Geometry check sheet. Reference: the model listing, model coordinates, mm. Face numbers are marked on the shaded views. A direction names the side the tool comes from. Coordinates: 2 decimals unless noted, no trailing zeros. Write each loop counter-clockwise with the first axis right and the second up, starting at its lowest first coordinate (ties: lowest second). Pieces come first, ordered by that corner, then holes. Notation, with made-up numbers: M 23,-30 L 62,-30 A22 ccw 62,-5 Z; hole C -27.75,45.5 d4. An arc over 180 degrees is marked long. Answer as a JSON object with one key per item and string values. Group by question number.
```python
from build123d import *

# Parameters (mm, degrees)
SKETCH_1_W          = 50
SKETCH_1_H          = 45
SKETCH_1_W_2        = 45
SKETCH_1_H_2        = 40
EXTRUDE_1_DEPTH     = 90
SKETCH_2_W          = 48.4
SKETCH_2_H          = 1.9
CUT_EXTRUDE_1_DEPTH = 36
SKETCH_3_R          = 13.5
CUT_EXTRUDE_2_DEPTH = 2.5
EXTRUDE_2_DEPTH     = 36
SKETCH_5_W          = 45
SKETCH_5_H          = 36
CUT_EXTRUDE_3_DEPTH = 50.2
CUT_EXTRUDE_4_DEPTH = 36
SKETCH_7_W          = 2.2
SKETCH_7_H          = 1.9
EXTRUDE_3_DEPTH     = 30
CHAMFER_1_SIZE      = 2.2
SKETCH_8_W          = 3.95
SKETCH_8_H          = 3.95
EXTRUDE_4_DEPTH     = 6
SKETCH_9_R          = 2.025
CUT_EXTRUDE_5_DEPTH = 5
SKETCH_10_W         = 3.95
SKETCH_10_H         = 5
SKETCH_10_H_2       = 7.5
SKETCH_10_H_3       = 3.95
EXTRUDE_5_DEPTH     = 6
CUT_EXTRUDE_START   = -5
SKETCH_11_R         = 2.025
CUT_EXTRUDE_6_DEPTH = 5
CHAMFER_2_SIZE      = 3.95
FILLET_1_R          = 1.2
CUT_EXTRUDE_7_REACH = 125.637


with BuildPart() as part:
    # 草圖1 → 填料-伸長1 (new body)
    with BuildSketch(Plane(origin=(0, 0, 0), x_dir=(1, 0, 0), z_dir=(0, 1, 0))):
        Rectangle(SKETCH_1_W, SKETCH_1_H)
        Rectangle(SKETCH_1_W_2, SKETCH_1_H_2, mode=Mode.SUBTRACT)
    extrude(amount=-EXTRUDE_1_DEPTH)

    # 草圖2 → 除料-伸長1 (cut)
    with BuildSketch(Plane(origin=(0, 0, 0), x_dir=(1, 0, 0), z_dir=(0, 1, 0))):
        with Locations((0, -14.05)):
            Rectangle(SKETCH_2_W, SKETCH_2_H)
    extrude(amount=-CUT_EXTRUDE_1_DEPTH, mode=Mode.SUBTRACT)

    # 草圖3 → 除料-伸長2 (cut)
    with BuildSketch(Plane.XY.offset(22.5)):
        with BuildLine():
            Line((-22.5, 0), (-22.5, -17.3))
            ThreePointArc((-22.5, -17.3), (-9, -3.8), (4.5, -17.3))
            Line((4.5, -17.3), (4.5, 0))
            Line((4.5, 0), (-22.5, 0))
        make_face()
        with Locations((-9, -17.3)):
            Circle(SKETCH_3_R)
    extrude(amount=-CUT_EXTRUDE_2_DEPTH, mode=Mode.SUBTRACT)

    # 草圖4 → 填料-伸長2 (add)
    with BuildSketch(Plane.XY.offset(22.5)):
        with BuildLine():
            Line((11, 0), (11, -17.3))
            ThreePointArc((11, -17.3), (5.142135624, -31.442135624), (-9, -37.3))
            Line((-9, -37.3), (-25, -37.3))
            Line((-25, -37.3), (-25, -90))
            Line((-25, -90), (25, -90))
            Line((25, -90), (25, 0))
            Line((25, 0), (11, 0))
        make_face()
    extrude(amount=EXTRUDE_2_DEPTH)

    # 草圖5 → 除料-伸長3 (cut)
    with BuildSketch(Plane(origin=(-25, -90, 58.5), x_dir=(1, 0, 0), z_dir=(0, -1, 0))):
        with Locations((25, -20.5)):
            Rectangle(SKETCH_5_W, SKETCH_5_H)
    extrude(amount=-CUT_EXTRUDE_3_DEPTH, mode=Mode.SUBTRACT)

    # 草圖6 → 除料-伸長4 (cut)
    with BuildSketch(Plane(origin=(0, 0, 20), x_dir=(-1, 0, 0), z_dir=(0, 0, -1))):
        with BuildLine():
            Line((-22.5, -2.5), (-22.5, -39.8))
            Line((-22.5, -39.8), (9, -39.8))
            ThreePointArc((9, -39.8), (-6.909902577, -33.209902577), (-13.5, -17.3))
            Line((-13.5, -17.3), (-13.5, -2.5))
            Line((-13.5, -2.5), (-22.5, -2.5))
        make_face()
    extrude(amount=-CUT_EXTRUDE_4_DEPTH, mode=Mode.SUBTRACT)

    # 草圖7 → 填料-伸長3 (add)
    with BuildSketch(Plane(origin=(0, -38.5, 0), x_dir=(1, 0, 0), z_dir=(0, 1, 0))):
        with Locations((-21.4, -14.05)):
            Rectangle(SKETCH_7_W, SKETCH_7_H)
    extrude(amount=-EXTRUDE_3_DEPTH)

    # 導角1
    chamfer_1_edges = [part.edges().sort_by_distance(p)[0] for p in [
        (-20.3, -38.5, 14.05),
        (-20.3, -68.5, 14.05),
    ]]
    chamfer(chamfer_1_edges, length=CHAMFER_1_SIZE - 0.0001)  # a hair under: the kernel refuses the full size

    # 草圖8 → 填料-伸長4 (add)
    with BuildSketch(Plane.XZ.offset(90)):
        with Locations((-20.525, 54.025)):
            Rectangle(SKETCH_8_W, SKETCH_8_H)
        with Locations((20.525, 54.025)):
            Rectangle(SKETCH_8_W, SKETCH_8_H)
        with Locations((20.525, -18.025)):
            Rectangle(SKETCH_8_W, SKETCH_8_H)
        with Locations((-20.525, -18.025)):
            Rectangle(SKETCH_8_W, SKETCH_8_H)
    extrude(amount=-EXTRUDE_4_DEPTH)

    # 草圖9 → 除料-伸長5 (cut)
    with BuildSketch(Plane.XZ.offset(90)):
        with Locations(Location((-21.775, 55.275, 0), (0, 0, 270))):
            Circle(SKETCH_9_R)
        with Locations(Location((21.775, 55.275, 0), (0, 0, 270))):
            Circle(SKETCH_9_R)
        with Locations(Location((-21.775, -19.275, 0), (0, 0, 270))):
            Circle(SKETCH_9_R)
        with Locations(Location((21.775, -19.275, 0), (0, 0, 270))):
            Circle(SKETCH_9_R)
    extrude(amount=-CUT_EXTRUDE_5_DEPTH, mode=Mode.SUBTRACT)

    # 草圖10 → 填料-伸長5 (add)
    with BuildSketch(Plane(origin=(0, 0, 0), x_dir=(1, 0, 0), z_dir=(0, 1, 0))):
        with Locations((20.525, -17.5)):
            Rectangle(SKETCH_10_W, SKETCH_10_H)
        with Locations((-20.525, -18.75)):
            Rectangle(SKETCH_10_W, SKETCH_10_H_2)
        with Locations((-20.525, 18.025)):
            Rectangle(SKETCH_10_W, SKETCH_10_H_3)
        with Locations((20.525, 18.025)):
            Rectangle(SKETCH_10_W, SKETCH_10_H_3)
    extrude(amount=-EXTRUDE_5_DEPTH)

    # 草圖11 → 除料-伸長6 (cut)
    with BuildSketch(Plane(origin=(0, 0, 0), x_dir=(1, 0, 0), z_dir=(0, 1, 0)).offset(CUT_EXTRUDE_START)):
        with Locations(Location((21.775, -18.225, 0), (0, 0, 270))):
            Circle(SKETCH_11_R)
        with Locations(Location((-21.775, -18.225, 0), (0, 0, 270))):
            Circle(SKETCH_11_R)
        with Locations(Location((21.775, 19.275, 0), (0, 0, 90))):
            Circle(SKETCH_11_R)
        with Locations(Location((-21.775, 19.275, 0), (0, 0, 90))):
            Circle(SKETCH_11_R)
    extrude(amount=CUT_EXTRUDE_6_DEPTH, mode=Mode.SUBTRACT)

    # 導角2
    chamfer_2_edges = [part.edges().sort_by_distance(p)[0] for p in [
        (-22.5, -6, 18.75),
        (22.5, -6, 17.5),
        (22.5, -6, -18.025),
        (-22.5, -6, -18.025),
    ]]
    chamfer(chamfer_2_edges, length=CHAMFER_2_SIZE - 0.0001)  # a hair under: the kernel refuses the full size

    # 圓角1
    fillet_1_edges = [part.edges().sort_by_distance(p)[0] for p in [
        (-18.55, -87, 52.05),
        (18.55, -87, 52.05),
        (18.55, -87, -16.05),
        (-18.55, -87, -16.05),
        (-18.55, -3, 15),
        (18.55, -3, 15),
        (-18.55, -3, -16.05),
        (18.55, -3, -16.05),
        (-25, -45, -22.5),
        (-25, -63.65, 58.5),
        (25, -45, 58.5),
        (25, -45, -22.5),
    ]]
    fillet(fillet_1_edges, radius=FILLET_1_R)

    # 草圖12 → 除料-伸長7 (cut, up to next)
    with BuildSketch(Plane.XY.offset(58.5), mode=Mode.PRIVATE) as cut_extrude_7_sk1:
        with BuildLine():
            Line((-2, -49.3), (-2, -45.672281323))
            ThreePointArc((-2, -45.672281323), (0, -39.3), (2, -45.672281323))
            Line((2, -45.672281323), (2, -49.3))
            ThreePointArc((2, -49.3), (0, -51.3), (-2, -49.3))
        make_face()
    cut_extrude_7_tool1 = extrude(cut_extrude_7_sk1.sketch, amount=-CUT_EXTRUDE_7_REACH, mode=Mode.PRIVATE) & part.part
    # 草圖12 → 除料-伸長7 (cut, up to next)
    with BuildSketch(Plane.XY.offset(58.5), mode=Mode.PRIVATE) as cut_extrude_7_sk2:
        with BuildLine():
            Line((-2, -84), (-2, -80.372281323))
            ThreePointArc((-2, -80.372281323), (0, -74), (2, -80.372281323))
            Line((2, -80.372281323), (2, -84))
            ThreePointArc((2, -84), (0, -86), (-2, -84))
        make_face()
    cut_extrude_7_tool2 = extrude(cut_extrude_7_sk2.sketch, amount=-CUT_EXTRUDE_7_REACH, mode=Mode.PRIVATE) & part.part
    add(cut_extrude_7_tool1.solids().sort_by_distance((0, -44.69051, 58.5))[0], mode=Mode.SUBTRACT)
    add(cut_extrude_7_tool2.solids().sort_by_distance((0, -79.39051, 58.5))[0], mode=Mode.SUBTRACT)


solid = part.part
```
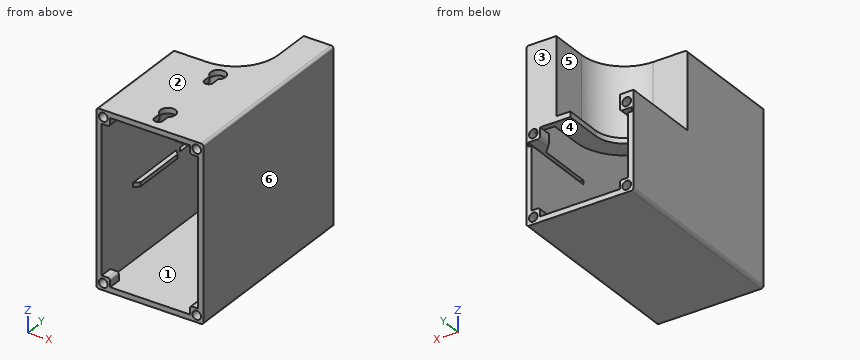
1) Section check C-C (y = -77.5). Record the cut outline in (x, z).
2) Material ranges on probe 1 along X at (y, z) = (-66.5, 27); probe 2 along Z at (x, y) = (6.5, -79); probe 3 along Z at (x, y) = (-13, -37), recorded low to high. Write a range as [from, to].
3) Section check D-D (y = -63). Record the cut outline in (x, z).
4) Set-up check for the marked faces 4, 5 and 6: record each of +Z, -Z, +X, -X, +Y, -Y from which the full face is reachable in a straight line by a thin tool's end or side.
5) Go/stop test with flat-tipped pins: pin 1 Ø4.5 at (x, z) = (-21.775, 55.275) entering from +Y; pin 2 Ø1.4 at (x, y) = (-21.5, -2.5) entering from +Z; pin 3 Ø6 at (x, z) = (-11, 47) entering from -Y. Record where each tip stops, or that it passes through.
6) Section check A-A (x = 17). Record the cut outline in (y, z).
7) Draft check along Z on the marked faces 1, 2 and 3. Enter one of: +Z half, -Z half, draft (parallel to the pull), parting line (faces both ways), or undercut.
8) Section check B-B (z = 5). Record the cut outline in (x, y).
Entries:
{
 "1": {"outline": "M -25,-21.3 A1.2 ccw -23.8,-22.5 L 23.8,-22.5 A1.2 ccw 25,-21.3 L 25,57.3 A1.2 ccw 23.8,58.5 L 3.5,58.5 L 3.5,56 L 22.5,56 L 22.5,-20 L -22.5,-20 L -22.5,56 L -3.5,56 L -3.5,58.5 L -23.8,58.5 A1.2 ccw -25,57.3 Z"},
 "2": {"probe 1": "[-25, -22.5], [22.5, 25]", "probe 2": "[-22.5, -20], [56, 58.5]", "probe 3": "[-22.5, -20], [20, 22.5]"},
 "3": {"outline": "M -25,-21.3 A1.2 ccw -23.8,-22.5 L 23.8,-22.5 A1.2 ccw 25,-21.3 L 25,57.3 A1.2 ccw 23.8,58.5 L -23.8,58.5 A1.2 ccw -25,57.3 Z; hole M -22.5,-20 L 22.5,-20 L 22.5,56 L -22.5,56 L -22.5,15 L -20.3,15 L -20.3,13.1 L -22.5,13.1 Z"},
 "4": {"face 4": "-Y", "face 5": "+Z, -X, +Y", "face 6": "+Z, -Z, +X, +Y, -Y"},
 "5": {"pin 1": "y = -37.3", "pin 2": "z = 22.5", "pin 3": "y = -39.8"},
 "6": {"outline": "M -90,-22.5 L 0,-22.5 L 0,-20 L -90,-20 Z; M -90,56 L -2.5,56 L -2.5,20 L 0,20 L 0,58.5 L -90,58.5 Z"},
 "7": {"face 1": "undercut", "face 2": "+Z half", "face 3": "draft"},
 "8": {"outline": "M -25,-90 L -22.5,-90 L -22.5,0 L -25,0 Z; M 22.5,-90 L 25,-90 L 25,0 L 22.5,0 Z"}
}
